```python
from build123d import *

# Parameters (mm, degrees)
SKETCH1_R                       = 11.1125
BOSS_EXTRUDE1_DEPTH             = 3.175
SKETCH2_R                       = 3.175
BOSS_EXTRUDE2_DEPTH             = 19.05
F_2_CLEARANCE_HOLE1_D           = 2.4384
SKETCH5_R                       = 1.984375
CUT_EXTRUDE1_DEPTH              = 1.5875
F_3_32_0_09375_DIAMETER_HOLE1_D = 2.38125


with BuildPart() as part:
    # Sketch1 → Boss-Extrude1 (new body)
    with BuildSketch(Plane(origin=(0, 0, 0), x_dir=(1, 0, 0), z_dir=(0, 1, 0))):
        with Locations(Location((0, 0, 0), (0, 0, 270))):
            Circle(SKETCH1_R)
    extrude(amount=BOSS_EXTRUDE1_DEPTH)

    # Sketch2 → Boss-Extrude2 (add)
    with BuildSketch(Plane(origin=(0, 3.175, 0), x_dir=(1, 0, 0), z_dir=(0, 1, 0))):
        with Locations(Location((0, 0, 0), (0, 0, 90))):
            Circle(SKETCH2_R)
    extrude(amount=BOSS_EXTRUDE2_DEPTH)

    # #2 Clearance Hole1 (through all)
    with Locations(Plane(origin=(0, 3.175, 0), x_dir=(1, 0, 0), z_dir=(0, 1, 0))):
        with Locations((0, -8), (0, 8), (-8, 0), (8, 0)):
            Hole(F_2_CLEARANCE_HOLE1_D / 2)

    # Sketch5 → Cut-Extrude1 (cut)
    with BuildSketch(Plane(origin=(0, 3.175, 0), x_dir=(1, 0, 0), z_dir=(0, 1, 0))):
        with Locations(Location((0, -8, 0), (0, 0, 270))):
            Circle(SKETCH5_R)
        with Locations(Location((8, 0, 0), (0, 0, 270))):
            Circle(SKETCH5_R)
        with Locations(Location((0, 8, 0), (0, 0, 270))):
            Circle(SKETCH5_R)
        with Locations(Location((-8, 0, 0), (0, 0, 270))):
            Circle(SKETCH5_R)
    extrude(amount=-CUT_EXTRUDE1_DEPTH, mode=Mode.SUBTRACT)

    # 3/32 (0.09375) Diameter Hole1 (through all)
    with Locations(Plane.XY.offset(3.175)):
        with Locations((0, 12.7)):
            Hole(F_3_32_0_09375_DIAMETER_HOLE1_D / 2)


solid = part.part
```
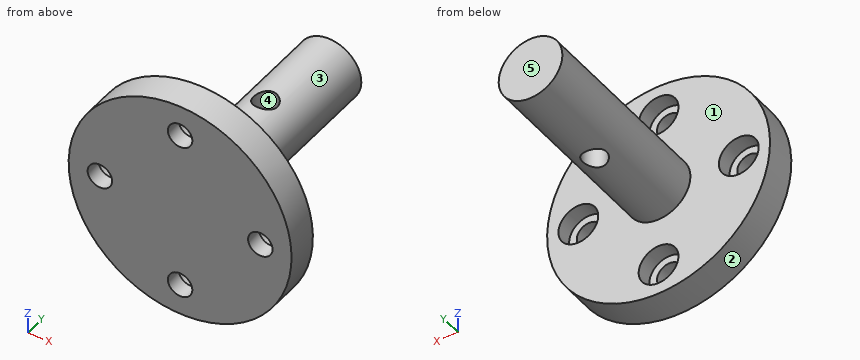
Build history of the part. All positions in model axes, mm. Face numbers are marked on the shaded views. A direction names the side the tool comes from. Give positions to 0.01 mm unless a question says otherwise; leave off trailing zeros. Order: outer loops, then holes, each group sorted by start corner. A loop starts at its lowest first (then second) coordinate and runs counter-clockwise, first axis right, second up. Notation, with made-up numbers: M 88.25,80 L 99.25,80 A8 cw 99.25,89 Z; hole C -21.75,60 d4. An arc over 180 degrees is marked long. Write item = value, one per line. Start each with the question number.
(1) Slice it at B-B on z = -8.75. Write the cut outline in (x, y) (1 decimal), plus the area to 3 significant figures.
(2) Which spindle directions (+Z, -Z, +X, -X, +Y, -Y) get a long thin tool onto all of the face, cutting with end or side? Do the marked faces 1 and 2. Say none if no direction does.
(3) Slice it at A-A on x = 8.75. Write the cut outline in (y, z) (1 decimal), plus the area to 3 significant figures.
(4) Pin check, flat tips, straight feed: pin 1 Ø3 at (x, y) = (0, 12.7) entering from -Z (3 decimals); pin 2 Ø3.5 at (x, z) = (8, 0) entering from +Y; pin 3 Ø4.5 at (x, z) = (0, 7.5) entering from +Y (3 decimals). Stop position of each tip, or through.
(5) Two-plate mould, pull along X, no slides. Class the marked faces 3, 4 and 5: released by +X, released by -X, zero draft, split by the parting line, or undercut.
(6) Slice it at D-D on y = 12.7. Write the cut outline in (x, z) (3 decimals), plus the area to 3 significant figures.
(7) Slice it at C-C on y = 15.75. Write the cut outline in (x, z) (3 decimals), plus the area to 3 significant figures.
(8) Probe L1, parallel to X at y = 2.1, z = 0; L2, parallel to Y at x = 0, z = -0.75 (3 decimals); L3, parallel to Z at x = -1.25, y = 3. List the from-to ranges inside material, lowest first. Write a range as [from, to].
Responses:
q1.outline = M -6.9,0 L -1,0 L -1,1.6 L -1.8,1.6 L -1.8,3.2 L -6.9,3.2 Z; M 1,0 L 6.9,0 L 6.9,3.2 L 1.8,3.2 L 1.8,1.6 L 1,1.6 Z
q1.area = 34.6 mm2
q2.face_1 = +Y
q2.face_2 = +Y, -Y
q3.outline = M 0,-6.9 L 3.2,-6.9 L 3.2,-1.8 L 1.6,-1.8 L 1.6,-1 L 0,-1 Z; M 0,1 L 1.6,1 L 1.6,1.8 L 3.2,1.8 L 3.2,6.9 L 0,6.9 Z
q3.area = 34.6 mm2
q4.pin_1 = -3.175
q4.pin_2 = 1.59
q4.pin_3 = 3.175
q5.face_3 = split by the parting line
q5.face_4 = undercut
q5.face_5 = zero draft
q6.outline = M -1.191,-2.943 L -1.191,2.943 A3.175 ccw Z; M 1.191,-2.943 A3.175 ccw 1.191,2.943 Z
q6.area = 16.9 mm2
q7.outline = C 0,0 d6.35
q7.area = 31.7 mm2
q8.L1 = [-11.11, -9.98], [-6.02, 6.02], [9.98, 11.11]
q8.L2 = [0, 11.509], [13.891, 22.225]
q8.L3 = [-11.04, -9.54], [-6.46, 6.46], [9.54, 11.04]
